```python
from build123d import *

# Parameters (mm, degrees)
SKETCH1_W           = 204.7875
SKETCH1_H           = 124.61875
BOSS_EXTRUDE1_DEPTH = 1.5875
EXTRUDE_THIN1_DEPTH = 14.2875
CUT_EXTRUDE1_DEPTH  = 165.658404983


with BuildPart() as part:
    # Sketch1 → Boss-Extrude1 (new body)
    with BuildSketch(Plane.XY):
        Rectangle(SKETCH1_W, SKETCH1_H)
    extrude(amount=BOSS_EXTRUDE1_DEPTH)

    # Sketch2 → Extrude-Thin1 (add)
    with BuildSketch(Plane(origin=(96.04375, 0, 0), x_dir=(0, 0, -1), z_dir=(1, 0, 0))):
        with BuildLine():
            Line((-1.04775, -62.309375), (-1.04775, -65.484375))
            ThreePointArc((-1.04775, -65.484375), (-0.74087113, -66.22524613), (0, -66.532125))
            Line((0, -66.532125), (4.22275, -66.532125))
            ThreePointArc((4.22275, -66.532125), (4.96362113, -66.22524613), (5.2705, -65.484375))
            Line((5.2705, -65.484375), (5.2705, -27.384375))
            Line((5.2705, -27.384375), (4.7625, -27.384375))
            Line((4.7625, -27.384375), (4.7625, -65.484375))
            ThreePointArc((4.7625, -65.484375), (4.604410885, -65.866035885), (4.22275, -66.024125))
            Line((4.22275, -66.024125), (0, -66.024125))
            ThreePointArc((0, -66.024125), (-0.381660885, -65.866035885), (-0.53975, -65.484375))
            Line((-0.53975, -65.484375), (-0.53975, -62.309375))
            Line((-0.53975, -62.309375), (-1.04775, -62.309375))
        make_face()
    extrude(amount=-EXTRUDE_THIN1_DEPTH)

    # Sketch3 → Cut-Extrude1 (cut, through all)
    with BuildSketch(Plane.XZ.offset(66.532125)):
        Polygon((81.75625, 0), (86.51875, -4.22275), (86.51875, -5.2705), (81.75625, -5.2705), align=None)
        Polygon((91.28125, -4.22275), (91.28125, -5.2705), (96.04375, -5.2705), (96.04375, 0), align=None)
    extrude(amount=-CUT_EXTRUDE1_DEPTH, mode=Mode.SUBTRACT)


solid = part.part
```
Can you work these out from the model? Positions are in its coordinate system, mm. A direction names the side the tool comes from. Coordinates: 2 decimals unless noted, no trailing zeros. Write each loop counter-clockwise with the first axis right and the second up, starting at its lowest first coordinate (ties: lowest second). Pieces come first, ordered by that corner, then holes. Notation, with made-up numbers: M 38,84.5 L 57,84.5 A30 ccw 57,120.5 Z; hole C -26.75,50 d7. An arc over 180 degrees is marked long. Answer as CSV lines item,"result".
Item 1: Imagine slicing it at B-B on y = -20.5. List the corners of the cut face in (x, z) for me.
Geometry results:
outline,"M -102.39,0 L 102.39,0 L 102.39,1.59 L -102.39,1.59 Z"
Item 2: I'm going to push flat-ended pins straight in: P1, Ø5, axis at x = -15, y = -36.5, coming from the -Z side; P2, Ø2, axis at x = 90, z = -2.5, coming from the +Y side; P3, Ø0.8, axis at y = -47.5, z = -4.5, coming from the +X side. Where does each tip first touch, or does it pass through?
Geometry results:
P1,"stops at z = 0"
P2,"stops at y = -66.02"
P3,"stops at x = 91.28"
Item 3: Please list where these lines run through material, in increasing order: line 1 along Y through (x, z) = (-50.5, 1.5); line 2 along Z through (x, y) = (-70.5, -30).
Geometry results:
line 1,"y = -62.31 to 62.31"
line 2,"z = 0 to 1.59"
Item 4: We'd pull the mould along Z, two halves only. Please class faces 3 (the flat face through (89, -66.532, -2)), 4 (the flat face through (89, -66.024, -2)), 5 (the flat face through (93.7, -66.28, -2.08)): +Z half, -Z half, draft (parallel to the pull), parting line (faces both ways), or undercut.
Geometry results:
face 3,"draft"
face 4,"undercut"
face 5,"-Z half"
Item 5: On a 3-axis mill with a long thin cutter (end or side, diameter ignored), from which of +Z, -Z, +X, -X, +Y, -Y can I reach the whole of each face in a straight line? I mean faces 1 (the flat face through (89, -46, -4.762)), 2 (the flat face through (-1, 1, 1.588)). Say none if no direction works.
Geometry results:
face 1,"+X, -X, +Y"
face 2,"+Z, +X, -X, +Y, -Y"
Item 6: Imagine slicing it at A-A on y = -54.5. List the corners of the cut face in (x, z) for me.
Geometry results:
outline,"M -102.39,0 L 102.39,0 L 102.39,1.59 L -102.39,1.59 Z; M 86.52,-5.27 L 91.28,-5.27 L 91.28,-4.76 L 86.52,-4.76 Z"
Item 7: Imagine slicing it at C-C on x = -50.5. List the corners of the cut face in (y, z) for me.
Geometry results:
outline,"M -62.31,0 L 62.31,0 L 62.31,1.59 L -62.31,1.59 Z"
